Part model, mm, in its own coordinate system. A direction names the side the tool comes from. Coordinates: 2 decimals unless noted, no trailing zeros. Loops run counter-clockwise (first coordinate to the right, second up) from the corner with the lowest first, then second, coordinate; pieces in that order, holes last. Notation, with made-up numbers: M 12.25,58.5 L 46.25,58.5 A4 cw 46.25,65.5 Z; hole C 54,-16 d9. An arc over 180 degrees is marked long. Use a Markdown table: item, result. Add a question column.
1) Band-saw the part on B-B (x = 38.1). List the corners of the cut face in (y, z).
2) Band-saw the part on A-A (z = -10). List the corners of the cut face in (x, y), plus the area to 3 significant figures.
3) Wall check: probe 1 along Z at (x, y) = (116, 10.75); probe 2 along Y at (x, z) = (39.5, -15). Give the ranges that are in metal, low to high. Write a range as from..to.
4) Pin check, flat tip, straight feed: pin 1 Ø11.5 at (x, z) = (111, -15.5) entering from +Y. Stop position of the tip, or through.
5) Pull direction Z, two halves, no side cores. Call faces 1 (the flat face through (75, 6, -50.8)), 2 (the flat face through (75, 0, -26)), 3 (the cylindrical face through (114.55, 12.23, -42.32)): released by +Z, released by -Z, zero draft, split by the parting line, or undercut.
6) Band-saw the part on C-C (x = 72.5). List the corners of the cut face in (y, z).
7) Tool access for faces 4 (the flat face through (76.1, 9.75, -20.8)), 5 (the flat face through (75, 6, 0)): list every direction of +Z, -Z, +X, -X, +Y, -Y with a clear straight run to the whole face (end or side of a thin tool).
from build123d import *

# Parameters (mm, degrees)
SKETCH1_W            = 152.4
SKETCH1_H            = 50.8
BOSS_EXTRUDE1_DEPTH  = 12.7
CUT_EXTRUDE1_DEPTH   = 0.95
CUT_EXTRUDE2_DEPTH   = 2
SKETCH4_R            = 5.5
BOSS_EXTRUDE2_DEPTH  = 2.95
LPATTERN1_COUNT      = 2
LPATTERN1_PITCH      = 38.1
LPATTERN1_COUNT_DIR2 = 2
LPATTERN1_PITCH_DIR2 = 38.1


with BuildPart() as part:
    # Sketch1 → Boss-Extrude1 (new body)
    with BuildSketch(Plane(origin=(0, 0, 0), x_dir=(1, 0, 0), z_dir=(0, 1, 0))):
        with Locations((76.2, 25.4)):
            Rectangle(SKETCH1_W, SKETCH1_H)
    extrude(amount=BOSS_EXTRUDE1_DEPTH)

    # Sketch2 → Cut-Extrude1 (cut)
    with BuildSketch(Plane(origin=(0, 12.7, 0), x_dir=(1, 0, 0), z_dir=(0, 1, 0))):
        with BuildLine():
            Line((64.626998, 30.75), (64.626998, 6.35))
            Line((64.626998, 6.35), (87.773002, 6.35))
            Line((87.773002, 6.35), (87.773002, 30.75))
            ThreePointArc((87.773002, 30.75), (76.2, 42.323002), (64.626998, 30.75))
        make_face()
    cut_extrude1 = extrude(amount=-CUT_EXTRUDE1_DEPTH, mode=Mode.SUBTRACT)

    # Sketch3 → Cut-Extrude2 (cut)
    with BuildSketch(Plane(origin=(0, 11.75, 0), x_dir=(1, 0, 0), z_dir=(0, 1, 0))):
        with BuildLine():
            Line((65.626998, 30.75), (65.626998, 7.35))
            Line((65.626998, 7.35), (86.773002, 7.35))
            Line((86.773002, 7.35), (86.773002, 30.75))
            ThreePointArc((86.773002, 30.75), (76.2, 41.323002), (65.626998, 30.75))
        make_face()
    cut_extrude2 = extrude(amount=-CUT_EXTRUDE2_DEPTH, mode=Mode.SUBTRACT)

    # Sketch4 → Boss-Extrude2 (add)
    with BuildSketch(Plane(origin=(0, 9.75, 0), x_dir=(1, 0, 0), z_dir=(0, 1, 0))):
        with Locations(Location((76.2, 26.6, 0), (0, 0, 90))):
            Circle(SKETCH4_R)
    boss_extrude2 = extrude(amount=BOSS_EXTRUDE2_DEPTH)

    # LPattern1: Cut-Extrude1, Cut-Extrude2, Boss-Extrude2 2 × 2
    with Locations(*[Vector(1, 0, 0) * (i * LPATTERN1_PITCH) + Vector(-1, 0, 0) * (j * LPATTERN1_PITCH_DIR2) for i in range(LPATTERN1_COUNT) for j in range(LPATTERN1_COUNT_DIR2) if (i, j) != (0, 0)]):
        add(cut_extrude1, mode=Mode.SUBTRACT)
        add(cut_extrude2, mode=Mode.SUBTRACT)
        add(boss_extrude2)


solid = part.part
Entries:
| question | item | result |
|---|---|---|
| 1 | outline | M 0,-50.8 L 12.7,-50.8 L 12.7,-42.32 L 11.75,-42.32 L 11.75,-41.32 L 9.75,-41.32 L 9.75,-32.1 L 12.7,-32.1 L 12.7,-21.1 L 9.75,-21.1 L 9.75,-7.35 L 11.75,-7.35 L 11.75,-6.35 L 12.7,-6.35 L 12.7,0 L 0,0 Z |
| 2 | outline | M 0,0 L 152.4,0 L 152.4,12.7 L 125.87,12.7 L 125.87,11.75 L 124.87,11.75 L 124.87,9.75 L 103.73,9.75 L 103.73,11.75 L 102.73,11.75 L 102.73,12.7 L 87.77,12.7 L 87.77,11.75 L 86.77,11.75 L 86.77,9.75 L 65.63,9.75 L 65.63,11.75 L 64.63,11.75 L 64.63,12.7 L 49.67,12.7 L 49.67,11.75 L 48.67,11.75 L 48.67,9.75 L 27.53,9.75 L 27.53,11.75 L 26.53,11.75 L 26.53,12.7 L 0,12.7 Z |
| 2 | area | 1,740 mm2 |
| 3 | probe 1 | -50.8..-41.19, -31.83..-21.37, -7.35..0 |
| 3 | probe 2 | 0..9.75 |
| 4 | pin 1 | y = 9.75 |
| 5 | face 1 | released by -Z |
| 5 | face 2 | zero draft |
| 5 | face 3 | undercut |
| 6 | outline | M 0,-50.8 L 12.7,-50.8 L 12.7,-41.72 L 11.75,-41.72 L 11.75,-40.65 L 9.75,-40.65 L 9.75,-30.67 L 12.7,-30.67 L 12.7,-22.53 L 9.75,-22.53 L 9.75,-7.35 L 11.75,-7.35 L 11.75,-6.35 L 12.7,-6.35 L 12.7,0 L 0,0 Z |
| 7 | face 4 | +Y |
| 7 | face 5 | +Z, +X, -X, +Y, -Y |
